Verification items for this drawing (mm, ordinates from the low corner). A direction names the side the tool comes from. Coordinates: 2 decimals unless noted, no trailing zeros. Loops run counter-clockwise (first coordinate to the right, second up) from the corner with the lowest first, then second, coordinate; pieces in that order, holes last. Notation, with made-up numbers: M 78,77 L 100,77 A20 cw 100,111 Z; hole C 35.5,-32.75 d3. An arc over 180 degrees is marked long. Use CSV: the item, a comma, the result in double quotes.
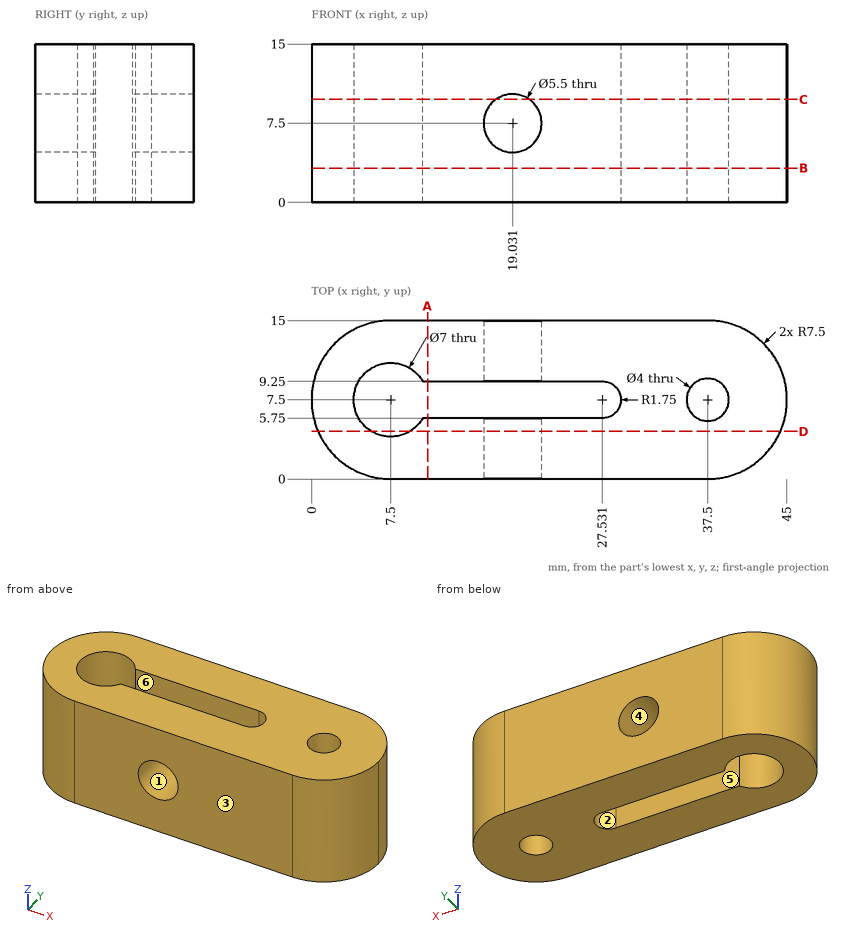
1. Section check C-C, the plane z = 9.75. Record the cut outline in (x, y).
The answers:
outline,"M 7.5,0 L 17.45,0 L 17.45,5.75 L 10.53,5.75 A3.5 cw long 10.53,9.25 L 17.45,9.25 L 17.45,15 L 7.5,15 A7.5 ccw Z; M 20.61,0 L 37.5,0 A7.5 ccw 37.5,15 L 20.61,15 L 20.61,9.25 L 27.53,9.25 A1.75 cw 27.53,5.75 L 20.61,5.75 Z; hole C 37.5,7.5 d4"
2. Thickness scan on line 1 (Y direction, x = 18, z = 2.5); line 2 (X direction, y = 6.75, z = 8.5); line 3 (Z direction, x = 18.5, y = 10.75). Record the ranges inside material, lowest first. Write a range as [from, to].
The answers:
line 1,"[0, 5.75], [9.25, 15]"
line 2,"[0.04, 4.08], [29.11, 35.65], [39.35, 44.96]"
line 3,"[0, 4.8], [10.2, 15]"
3. Set-up check for the marked faces 1 and 2: record each of +Z, -Z, +X, -X, +Y, -Y from which the full face is reachable in a straight line by a thin tool's end or side.
The answers:
face 1,"+Y, -Y"
face 2,"+Z, -Z"
4. Section check A-A, the plane x = 11. Record the cut outline in (y, z), plus the area to 4 significant figures.
The answers:
outline,"M 0,0 L 5.75,0 L 5.75,15 L 0,15 Z; M 9.25,0 L 15,0 L 15,15 L 9.25,15 Z"
area,"172.5 mm^2"
5. Gauge pin test, flat ends, axial feed: P1, Ø5, axis at y = 2.5, z = 6, coming from the +X side; P2, Ø3, axis at y = 4.5, z = 12, coming from the +X side. Record the tip position at first contact, or that the pin passes through.
The answers:
P1,"x = 44.57"
P2,"x = 44.85"
6. Section check D-D, the plane y = 4.5. Record the cut outline in (x, z).
The answers:
outline,"M 0.63,0 L 5.7,0 L 5.7,15 L 0.63,15 Z; M 9.3,0 L 44.37,0 L 44.37,15 L 9.3,15 Z; hole C 19.03,7.5 d5.5"
7. Section check B-B, the plane z = 3.25. Record the cut outline in (x, y).
The answers:
outline,"M 7.5,0 L 37.5,0 A7.5 ccw 37.5,15 L 7.5,15 A7.5 ccw Z; hole M 10.53,5.75 L 27.53,5.75 A1.75 ccw 27.53,9.25 L 10.53,9.25 A3.5 ccw long Z; hole C 37.5,7.5 d4"
8. Release check for a two-part mould opening along Y. For the marked faces 3, 4, 5 and 6 record: +Y half, -Y half, draft (parallel to the pull), parting line (faces both ways), or undercut.
The answers:
face 3,"-Y half"
face 4,"draft"
face 5,"undercut"
face 6,"undercut"
